Work out the finished part from the listing and answer in its coordinate system (mm). Face numbers are marked on the shaded views. Round coordinates to 2 decimals unless told otherwise and drop trailing zeros. Order: outer loops, then holes, each group sorted by start corner. A loop starts at its lowest first (then second) coordinate and runs counter-clockwise, first axis right, second up. Notation, with made-up numbers: (-31.5, -37.75) - (14.5, -37.75) arc R20 ccw to (14.5, -10.75) - close; hole circle Ø10 at (42, 9). An arc over 180 degrees is marked (long way). Use one line per item in the form item = value. Start each with the question number.
Q1. The part is cut by section D-D on y = -126. Determine the outline of the cut face in (x, z), plus the area to 3 significant figures.
Q2. The part is cut by section B-B on x = 563. Determine the outline of the cut face in (y, z), plus the area to 3 significant figures.
Q3. The part is cut by section C-C on z = -85.5. Determine the outline of the cut face in (x, y).
Q4. Given P1, Ø14.5, axis at x = 697, z = 4, coming from the -Y side; P2, Ø6, axis at x = 903.5, z = -152, coming from the +Y side; P3, Ø12.5, axis at y = -65, z = 2, coming from the +X side, each flat-ended and moving along its own axis, determine where each tip first touches the part or whether it passes through.
Q5. The part is cut by section A-A on y = -44.5. Determine the outline of the cut face in (x, z), plus the area to 3 significant figures.
Q6. Find the intervals of material crossed by line 1 (Y direction, x = 796, z = -10); line 2 (Z direction, x = 720, y = -85.5) (3 decimals); line 3 (Y direction, x = 576.5, z = -188.5), in increasing order. Write a range as [from, to].
Q7. For a pull along Y with two mould halves and no side action, classify the marked faces 1 and 2 as +Y half, -Y half, draft (parallel to the pull), parting line (faces both ways), or undercut.
from build123d import *

# Parameters (mm, degrees)
F1_DEPTH      = 19.05
F2_W          = 355.6
F2_H          = 66.675
F2_W_2        = 101.6
F2_W_3        = 165.1
F2_H_2        = 76.2000030398
F3_DEPTH      = 19.05
F4_W          = 101.6
F4_H          = 19.05
F4_W_2        = 355.6
F4_W_3        = 165.1
F5_DEPTH      = 15.875
F6_W          = 241.3
F6_H          = 152.4
F7_DEPTH      = 19.05
F8_W          = 241.3
F8_H          = 19.05
F8_W_2        = 152.4
F9_DEPTH      = 38.1
F10_DEPTH     = 12.7
F11_T1_DEPTH  = 51.7103739472
F11_T3_DEPTH  = 51.7103739472
F11_T5_DEPTH  = 51.7103739472
F11_T7_DEPTH  = 51.7103739472
F11_T9_DEPTH  = 51.7103739472
F11_T11_DEPTH = 42.3922386312


# Not quite as in the source:
# - a fillet or chamfer that OpenCascade refuses, or shapes differently, is made with other operations: its cross-section is extruded or revolved along the edge and cut away or added
# - ends of sketch curves that miss each other by under 0.0002 mm in the source are joined


with BuildPart() as f1:
    # F0 (on Front) → F1 (new body)
    with BuildSketch(Plane.XZ):
        Polygon((1219.2, 0), (0, 0), (0, -215.9), (762, -215.9), (1219.2, -50.8), align=None)
    extrude(amount=F1_DEPTH)

    # F2 (on face) → F3 (join)
    with BuildSketch(Plane.XY):
        with Locations((177.8, 14.2875)):
            Rectangle(F2_W, F2_H)
        with Locations((1168.4, 14.2875)):
            Rectangle(F2_W_2, F2_H)
        with Locations((717.55, -57.1500015199)):
            Rectangle(F2_W_3, F2_H_2)
        Polygon((635, 0), (635, -19.05), (800.1, -19.05), (800.1, -3.0398e-06), (647.7, 0), align=None)
    extrude(amount=F3_DEPTH)

    # F4 (on face) → F5 (join)
    with BuildSketch(Plane.XY):
        with Locations((1168.4, 38.1)):
            Rectangle(F4_W, F4_H)
        with Locations((177.8, 38.1)):
            Rectangle(F4_W_2, F4_H)
        with Locations((717.55, -85.7250030398)):
            Rectangle(F4_W_3, F4_H)
    extrude(amount=-F5_DEPTH)

    # F6 (on face) → F7 (join)
    with BuildSketch(Plane(origin=(0, 0, -215.9), x_dir=(1, 0, 0), z_dir=(0, 0, -1))):
        Polygon((0, 95.25), (0, 0), (762, 0), (762, 95.25), (241.3, 95.25), align=None)
        with Locations((120.65, 171.45)):
            Rectangle(F6_W, F6_H)
    extrude(amount=F7_DEPTH)

    # F8 (on face) → F9 (join)
    with BuildSketch(Plane.XY.offset(-215.9)):
        with Locations((120.65, -238.125)):
            Rectangle(F8_W, F8_H)
        with Locations((330.2, -85.725)):
            Rectangle(F8_W_2, F8_H)
    extrude(amount=F9_DEPTH)

    # F10 (add): a face of the model
    f10_faces = [f1.faces().sort_by_distance(p)[0] for p in [
        (717.55, -85.7250030398, -15.875),
    ]]
    extrude(f10_faces, amount=F10_DEPTH)

    # F11: chamfer of 6.35 on 12 edges, made by hand

    # F11_s2 → F11_t1 (cut)
    with BuildSketch(Plane.XZ.offset(212.2698130264)):
        Polygon((6.35, -177.8), (0, -184.15), (0, -177.8), align=None)
        Polygon((241.3, -184.15), (234.95, -177.8), (241.3, -177.8), align=None)
    extrude(amount=F11_T1_DEPTH, mode=Mode.SUBTRACT)

    # F11_s4 → F11_t3 (cut)
    with BuildSketch(Plane.XZ.offset(59.8698130264)):
        Polygon((260.35, -177.8), (254, -184.15), (254, -177.8), align=None)
        Polygon((406.4, -184.15), (400.05, -177.8), (406.4, -177.8), align=None)
    extrude(amount=F11_T3_DEPTH, mode=Mode.SUBTRACT)

    # F11_s6 → F11_t5 (cut)
    with BuildSketch(Plane.XZ.offset(59.8698160663)):
        Polygon((800.1, -22.225), (793.75, -28.575), (800.1, -28.575), align=None)
        Polygon((635, -22.225), (641.35, -28.575), (635, -28.575), align=None)
    extrude(amount=F11_T5_DEPTH, mode=Mode.SUBTRACT)

    # F11_s8 → F11_t7 (cut)
    with BuildSketch(Plane.XY.offset(-251.2801869736)):
        Polygon((762, -88.9), (755.65, -95.25), (762, -95.25), align=None)
    extrude(amount=F11_T7_DEPTH, mode=Mode.SUBTRACT)

    # F11_s10 → F11_t9 (cut)
    with BuildSketch(Plane.XZ.offset(-63.9551869736)):
        Polygon((1219.2, -9.525), (1212.85, -15.875), (1219.2, -15.875), align=None)
        Polygon((355.6, -9.525), (349.25, -15.875), (355.6, -15.875), align=None)
        Polygon((1117.6, -9.525), (1123.95, -15.875), (1117.6, -15.875), align=None)
        Polygon((0, -9.525), (6.35, -15.875), (0, -15.875), align=None)
    extrude(amount=F11_T9_DEPTH, mode=Mode.SUBTRACT)

    # F11_s12 → F11_t11 (cut)
    with BuildSketch(Plane.XZ.offset(-11.6711193156)):
        Polygon((1219.2, -46.3417146679), (1215.006742345, -52.314231931), (1219.2, -50.8), align=None)
    extrude(amount=F11_T11_DEPTH, mode=Mode.SUBTRACT)


solid = f1.part
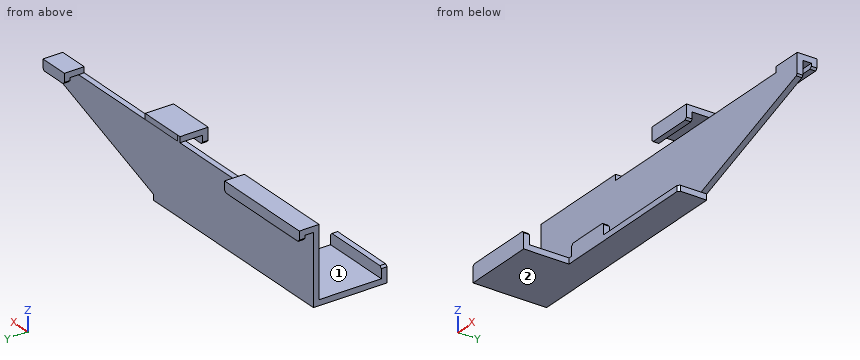
Found:
q1.outline = (0, -234.95) - (241.3, -234.95) - (241.3, -215.9) - (0, -215.9) - close
q1.area = 4,600 mm²
q2.outline = (-95.25, -234.95) - (0, -234.95) - (0, 0) - (-19.05, 0) - (-19.05, -215.9) - (-95.25, -215.9) - close
q2.area = 5,930 mm²
q3.outline = (0, -19.05) - (1123.11, -19.05) - (1123.11, 0) - (0, 0) - close
q4.P1 = -95.25
q4.P2 = 0
q4.P3 = 800.1
q5.outline = (0, -234.95) - (762, -234.95) - (762, -215.9) - (0, -215.9) - close; (635, 0) - (800.1, 0) - (800.1, 19.05) - (635, 19.05) - close
q5.area = 17,700 mm²
q6.line_1 = [-95.25, -76.2], [-19.05, 0]
q6.line_2 = [-234.95, -215.9], [-28.575, 19.05]
q6.line_3 = [-19.05, 0]
q7.face_1 = undercut
q7.face_2 = draft
